from build123d import *

# Parameters (mm, degrees)
SKETCH1_R           = 4.1
BOSS_EXTRUDE1_DEPTH = 30


with BuildPart() as part:
    # Sketch1 → Boss-Extrude1 (new body)
    with BuildSketch(Plane.XY):
        with BuildLine():
            ThreePointArc((2.121320344, 62.15218613), (0.128747602, 58.750955542), (0.053741668, 54.809751443))
            ThreePointArc((0.053741668, 54.809751443), (-0.804117699, 54.754085047), (-1.644372539, 54.572444612))
            ThreePointArc((-1.644372539, 54.572444612), (-2.072579341, 54.409614804), (-2.471000729, 54.183484289))
            ThreePointArc((-2.471000729, 54.183484289), (-3.749930813, 53.810707626), (-5.008263036, 54.248))
            ThreePointArc((-5.008263036, 54.248), (-6.975263036, 53.967), (-6.694263036, 52))
            ThreePointArc((-6.694263036, 52), (-5.044448782, 51.185750479), (-3.211825355, 51.023329036))
            ThreePointArc((-3.211825355, 51.023329036), (-2.346266102, 51.205491656), (-1.541903785, 51.573428203))
            ThreePointArc((-1.541903785, 51.573428203), (1.27066207, 51.717612537), (2.963447684, 49.46688095))
            ThreePointArc((2.963447684, 49.46688095), (5.265961581, 28.292845916), (4.96853298, 6.996065265))
            ThreePointArc((4.96853298, 6.996065265), (4.443724564, 6.189701484), (3.481666266, 6.199201562))
            ThreePointArc((3.481666266, 6.199201562), (-6.277419511, -3.338578183), (7.086411369, -0.578682913))
            ThreePointArc((7.086411369, -0.578682913), (7.189943669, 0.602744357), (7.307479638, 1.782860719))
            ThreePointArc((7.307479638, 1.782860719), (8.182981219, 25.916176913), (5.733322853, 49.940802351))
            ThreePointArc((5.733322853, 49.940802351), (5.169389034, 51.652077868), (4.108290399, 53.108290399))
            ThreePointArc((4.108290399, 53.108290399), (2.646753237, 56.636753237), (4.108290399, 60.165216075))
            ThreePointArc((4.108290399, 60.165216075), (4.108290399, 62.15218613), (2.121320344, 62.15218613))
        make_face()
        Circle(SKETCH1_R, mode=Mode.SUBTRACT)
    extrude(amount=BOSS_EXTRUDE1_DEPTH)


solid = part.part
Check sheet for the modelled part. Datum: model origin and axes. Units: mm. A direction names the side the tool comes from. Round coordinates to 2 decimals unless told otherwise and drop trailing zeros. Loops run counter-clockwise (first coordinate to the right, second up) from the corner with the lowest first, then second, coordinate; pieces in that order, holes last.
1. Sectioned sample at B-B on y = 56. Record the boundary of the cut face in (x, z).
2. Gauge pin test, flat ends, axial feed: pin 1 Ø10 at (y, z) = (0, 8) entering from -X; pin 2 Ø2 at (y, z) = (14, 7.5) entering from +X. Record the tip position at first contact, or that the pin passes through.
3. Set-up check for faces 1 (the cylindrical face through (4.46, 6.2, 14.79)), 2 (the flat face through (6, 25, 30)): record each of +Z, -Z, +X, -X, +Y, -Y from which the full face is reachable in a straight line by a thin tool's end or side.
4. Mould release check, pull along Y, two halves, no side actions. Record for faces 3 (the cylindrical face through (2.647, 56.582, 14.79)), 4 (the cylindrical face through (8.194, 25.578, 14.79)), 5 (the cylindrical face through (-3.73, 53.81, 14.79)), 6 (the flat face through (6, 25, 0)): released by +Y, released by -Y, zero draft, split by the parting line, or undercut.
5. Scan lines: probe 1 along Y at (x, z) = (-0.5, 3.75); probe 2 along Y at (x, z) = (-3.5, 18.25); probe 3 along X at (y, z) = (1.5, 20.25). Record each from-to range of solid material in increasing order.
6. Sectioned sample at A-A on z = 14. Record the boundary of the cut face in (x, y) (3 decimals), and give its area (3 significant figures).
Recorded:
1. outline: (-0.14, 0) - (2.69, 0) - (2.69, 30) - (-0.14, 30) - close
2. pin 1: stops at x = -7.11
2. pin 2: stops at x = 8.2
3. face 1: +Z, -Z
3. face 2: +Z, +X, -X, +Y, -Y
4. face 3: undercut
4. face 4: split by the parting line
4. face 5: released by +Y
4. face 6: zero draft
5. probe 1: y = -7.09 to -4.07, 4.07 to 7.09, 51.96 to 54.79
5. probe 2: y = -6.19 to -2.14, 2.14 to 6.19, 51 to 53.82
5. probe 3: x = -6.95 to -3.82, 3.82 to 7.28
6. outline: (-6.694, 52) arc R5 ccw to (-3.212, 51.023) arc R4 ccw to (-1.542, 51.573) arc R3 cw to (2.963, 49.467) arc R174.287 cw to (4.969, 6.996) arc R1 cw to (3.482, 6.199) arc R7.11 ccw (long way) to (7.086, -0.579) arc R100 cw to (7.307, 1.783) arc R175.291 ccw to (5.733, 49.941) arc R5.81 ccw to (4.108, 53.108) arc R4.99 cw to (4.108, 60.165) arc R1.405 ccw to (2.121, 62.152) arc R7.8 ccw to (0.054, 54.81) arc R5.81 ccw to (-1.644, 54.572) arc R3 ccw to (-2.471, 54.183) arc R2.19 cw to (-5.008, 54.248) arc R1.405 ccw to start; hole circle Ø8.2 at (0, 0)
6. area: 299 mm2
